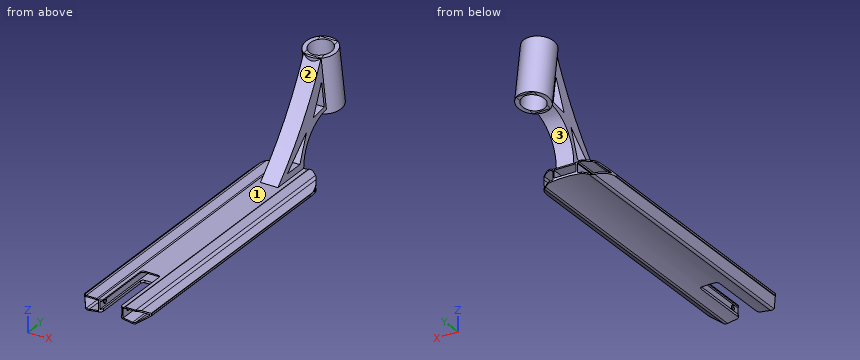
```python
from build123d import *

# Parameters (mm, degrees)
F1_DEPTH       = 250
F2_W           = 38
F2_H           = 13
F3_DEPTH       = 250
F4_T1_DEPTH    = 509.3674969976
F5_R           = 9
F6_R           = 1
F8_DEPTH       = 500.001
F10_DEPTH      = 24.4523840141
F10_DEPTH_BACK = 527
F12_DEPTH      = 527
F12_DEPTH_BACK = 24.4523841141
F13_F1_R       = 4.9999
F13_F2_R       = 4.9999
F13_F3_R       = 5
F13_F4_R       = 5
F13_F5_R       = 5
F13_F6_R       = 5
F15_DEPTH      = 15
F16_R          = 27.4590604355
F17_DEPTH      = 100
F19_D          = 40
F21_D          = 8
F21_DEPTH      = 50
F21_TIP        = 2.4034424761
F23_DEPTH      = 72.5010001


# Not quite as in the source:
# - a fillet or chamfer that OpenCascade refuses, or shapes differently, is made with other operations: its cross-section is extruded or revolved along the edge and cut away or added
# - a fillet or chamfer is up to 0.001 mm smaller than in the source, because OpenCascade refuses the exact size
# - an extrude ends at something that could not be found from the text; its depth is read off the source's solid


with BuildPart() as f1:
    # F0 (on Front) → F1 (new body, symmetric)
    with BuildSketch(Plane.XZ):
        with BuildLine():
            Line((22.5, 23.1513840141), (0, 23.1513840141))
            Line((0, 23.1513840141), (-22.5, 23.1513840141))
            Line((-22.5, 23.1513840141), (-22.5, 24.4513840141))
            Line((-22.5, 24.4513840141), (-45.5824640741, 24.4513840141))
            Line((-45.5824640741, 24.4513840141), (-57.5, 14.4513840141))
            Line((-57.5, 14.4513840141), (-57.5, 10.4513840141))
            Line((-57.5, 10.4513840141), (-40.1794919243, 0.4513840141))
            ThreePointArc((-40.1794919243, 0.4513840141), (0, 4.5289288725), (40.1794919243, 0.4513840141))
            Line((40.1794919243, 0.4513840141), (57.5, 10.4513840141))
            Line((57.5, 10.4513840141), (57.5, 14.4513840141))
            Line((57.5, 14.4513840141), (45.5824640741, 24.4513840141))
            Line((45.5824640741, 24.4513840141), (22.5, 24.4513840141))
            Line((22.5, 24.4513840141), (22.5, 23.1513840141))
        make_face()
    extrude(amount=F1_DEPTH, both=True)

    # F2 (on Front) → F3 (cut, symmetric)
    with BuildSketch(Plane.XZ):
        with Locations((0, 14.6513840141)):
            Rectangle(F2_W, F2_H)
    extrude(amount=F3_DEPTH, both=True, mode=Mode.SUBTRACT)

    # F4: fillet of radius 2 on 2 edges, made by hand

    # F4_s2 → F4_t1 (cut)
    with BuildSketch(Plane.XZ.offset(-254.6837484988)):
        with BuildLine():
            ThreePointArc((-24.3734993995, 24.4513840141), (-23.2333239744, 24.0945516866), (-22.5, 23.1513840141))
            Line((-22.5, 23.1513840141), (-22.5, 24.4513840141))
            Line((-22.5, 24.4513840141), (-24.3734993995, 24.4513840141))
        make_face()
        with BuildLine():
            ThreePointArc((24.3734993995, 24.4513840141), (23.2333239744, 24.0945516866), (22.5, 23.1513840141))
            Line((22.5, 23.1513840141), (22.5, 24.4513840141))
            Line((22.5, 24.4513840141), (24.3734993995, 24.4513840141))
        make_face()
    extrude(amount=F4_T1_DEPTH, mode=Mode.SUBTRACT)

    # F5
    f5_edges = [f1.edges().sort_by_distance(p)[0] for p in [
        (-45.582464, 0, 24.451384),
        (-40.179492, 0, 0.451384),
        (40.179492, 0, 0.451384),
        (45.582464, 0, 24.451384),
    ]]
    fillet(f5_edges, radius=F5_R)

    # F6
    f6_edges = [f1.edges().sort_by_distance(p)[0] for p in [
        (57.5, 0, 14.451384),
        (57.5, 0, 10.451384),
        (-57.5, 0, 10.451384),
        (-57.5, 0, 14.451384),
    ]]
    fillet(f6_edges, radius=F6_R)

    # F7 (on face) → F8 (cut, through all)
    with BuildSketch(Plane.XZ.offset(250)):
        with BuildLine():
            ThreePointArc((-42.1022690923, 3.8709010064), (-39.7790673433, 3.0327059534), (-37.3093701274, 3.0535140017))
            ThreePointArc((-37.3093701274, 3.0535140017), (-29.1789785809, 4.4103617496), (-21, 5.4343792715))
            Line((-21, 5.4343792715), (-21, 21.1513840141))
            Line((-21, 21.1513840141), (-22.5, 21.1513840141))
            ThreePointArc((-22.5, 21.1513840141), (-23.2333239744, 22.0945516866), (-24.3734993995, 22.4513840141))
            Line((-24.3734993995, 22.4513840141), (-42.3067319657, 22.4513840141))
            ThreePointArc((-42.3067319657, 22.4513840141), (-44.7008729689, 22.0292323596), (-46.8062452335, 20.813695116))
            Line((-46.8062452335, 20.813695116), (-55.7563117574, 13.3036975967))
            ThreePointArc((-55.7563117574, 13.3036975967), (-56.1097188459, 12.4504974108), (-55.6135241478, 11.6716277498))
            Line((-55.6135241478, 11.6716277498), (-42.1022690923, 3.8709010064))
        make_face()
        with BuildLine():
            Line((21, 21.1513840141), (21, 5.4343792715))
            ThreePointArc((21, 5.4343792715), (29.1789785809, 4.4103617496), (37.3093701274, 3.0535140017))
            ThreePointArc((37.3093701274, 3.0535140017), (39.7790673433, 3.0327059534), (42.1022690923, 3.8709010064))
            Line((42.1022690923, 3.8709010064), (55.6135241478, 11.6716277498))
            ThreePointArc((55.6135241478, 11.6716277498), (56.1097188459, 12.4504974108), (55.7563117574, 13.3036975967))
            Line((55.7563117574, 13.3036975967), (46.8062452335, 20.813695116))
            ThreePointArc((46.8062452335, 20.813695116), (44.7008729689, 22.0292323596), (42.3067319657, 22.4513840141))
            Line((42.3067319657, 22.4513840141), (24.3734993995, 22.4513840141))
            ThreePointArc((24.3734993995, 22.4513840141), (23.2333239744, 22.0945516866), (22.5, 21.1513840141))
            Line((22.5, 21.1513840141), (21, 21.1513840141))
        make_face()
    extrude(amount=-F8_DEPTH, mode=Mode.SUBTRACT)

    # F9 (on Top) → F10 (cut, two sides)
    with BuildSketch(Plane.XY) as f10_sk:
        with BuildLine():
            ThreePointArc((-57.5, 200), (0, 257.5), (57.5, 200))
            Line((57.5, 200), (57.5, 280))
            Line((57.5, 280), (-57.5, 280))
            Line((-57.5, 280), (-57.5, 200))
        make_face()
    extrude(amount=F10_DEPTH, mode=Mode.SUBTRACT)
    extrude(f10_sk.sketch, amount=-F10_DEPTH_BACK, mode=Mode.SUBTRACT)

    # F11 (on Top) → F12 (cut, two sides)
    with BuildSketch(Plane.XY) as f12_sk:
        Polygon((-43.2975540478, -250), (-68, -216), (-68, -346), (68, -346), (68, -216), (43.2975540478, -250), (16, -250), (16, -140), (-16, -140), (-16, -250), align=None)
    extrude(amount=-F12_DEPTH, mode=Mode.SUBTRACT)
    extrude(f12_sk.sketch, amount=F12_DEPTH_BACK, mode=Mode.SUBTRACT)

    # F13: fillet of radius 5 on 8 edges, made by hand

    # F13_f1 (radius 5 in the source; OpenCascade refuses exactly that, so slightly less here)
    f13_f1_edges = [f1.edges().sort_by_distance(p)[0] for p in [
        (-16, -250, 22.1513840141),
    ]]
    fillet(f13_f1_edges, radius=F13_F1_R)

    # F13_f2 (radius 5 in the source; OpenCascade refuses exactly that, so slightly less here)
    f13_f2_edges = [f1.edges().sort_by_distance(p)[0] for p in [
        (16, -250, 6.0196427984),
    ]]
    fillet(f13_f2_edges, radius=F13_F2_R)

    # F13_f3
    f13_f3_edges = [f1.edges().sort_by_distance(p)[0] for p in [
        (16, -140, 22.1513840141),
    ]]
    fillet(f13_f3_edges, radius=F13_F3_R)

    # F13_f4
    f13_f4_edges = [f1.edges().sort_by_distance(p)[0] for p in [
        (-16, -140, 22.1513840141),
    ]]
    fillet(f13_f4_edges, radius=F13_F4_R)

    # F13_f5
    f13_f5_edges = [f1.edges().sort_by_distance(p)[0] for p in [
        (-16, -140, 6.0196427984),
    ]]
    fillet(f13_f5_edges, radius=F13_F5_R)

    # F13_f6
    f13_f6_edges = [f1.edges().sort_by_distance(p)[0] for p in [
        (16, -140, 6.0196427984),
    ]]
    fillet(f13_f6_edges, radius=F13_F6_R)

    # F14 (on Right) → F15 (join, symmetric)
    with BuildSketch(Plane.YZ):
        with BuildLine():
            ThreePointArc((297.3819995028, 183.1513840141), (245.9666940414, 97.8136618671), (180, 23.1513840141))
            Line((180, 23.1513840141), (250, 23.1513840141))
            ThreePointArc((250, 23.1513840141), (267.6550746197, 69.6272787008), (311.7145367693, 92.6593051387))
            Line((311.7145367693, 92.6593051387), (313.0254460068, 84.3825499546))
            Line((313.0254460068, 84.3825499546), (358.4591096742, 91.5785353465))
            Line((358.4591096742, 91.5785353465), (342.8156631702, 190.347369406))
            Line((342.8156631702, 190.347369406), (297.3819995028, 183.1513840141))
        make_face()
    extrude(amount=F15_DEPTH, both=True)

    # F16 (on face) → F17 (join, through all)
    with BuildSketch(Plane(origin=(0, -21.0209895784, 132.7213047908), x_dir=(1, 0, 0), z_dir=(0, -0.156434465, 0.9876883406))):
        with Locations((0, 345.3719223914)):
            Circle(F16_R)
    extrude(amount=-F17_DEPTH)

    # F19 (through all)
    with Locations(Plane(origin=(0, -21.0209895784, 132.7213047908), x_dir=(1, 0, 0), z_dir=(0, -0.156434465, 0.9876883406))):
        with Locations((0, 345.3719223914)):
            Hole(F19_D / 2)

    # F21 (one way)
    with BuildSketch(Plane.YZ.offset(21)):
        with Locations((-236, 15.4343792715)):
            Circle(F21_D / 2)
    extrude(amount=-F21_DEPTH, mode=Mode.SUBTRACT)
    with Locations(Plane.YZ.offset(21)):
        with Locations((-236, 15.4343792715)):
            with Locations((0, 0, -(F21_DEPTH + F21_TIP / 2))):  # 118° drill point
                Cone(0, F21_D / 2, F21_TIP, mode=Mode.SUBTRACT)

    # F22 (on face) → F23 (cut, through all)
    with BuildSketch(Plane.YZ.offset(15)):
        Polygon((205.6868169308, 34.2114791274), (239.6868169308, 33.9609570801), (257.5687806787, 78.9609570801), align=None)
        Polygon((305.8015852264, 98.9295560122), (298.6742854118, 143.9295560122), (276.1709350086, 94.2365220609), align=None)
    extrude(amount=-F23_DEPTH, mode=Mode.SUBTRACT)


solid = f1.part
```
Source: CAD feature listing. Evaluate the final solid. Frame: model axes, mm. Face numbers are marked on the shaded views. Coordinates: 2 decimals unless noted, no trailing zeros. Loops run counter-clockwise (first coordinate to the right, second up) from the corner with the lowest first, then second, coordinate; pieces in that order, holes last. Notation, with made-up numbers: M 48.25,-35.5 L 79.25,-35.5 A23 cw 79.25,-6.5 Z; hole C -29.5,23.5 d8. An arc over 180 degrees is marked long. Use a Markdown table: item, result. Add a question column.
Q1. First-contact query: pin 1 (3 mm diameter, centred on y = 74, z = 23.5, fed in from +X); pin 2 (1.2 mm diameter, centred on x = 21.5, y = 78, fed in from -Z); pin 3 (5 mm diameter, centred on y = -236, z = 15.43, fed in from +X); pin 4 (17.5 mm diameter, centred on y = -34, z = 16.5, fed in from +X). Flat tips, straight axial feed; report the tip coordinate or a pass-through.
Q2. Material intervals for L1, parallel to Z at x = -20.2, y = -236; L2, parallel to Z at x = 30, y = 212; L3, parallel to Z at x = 14, y = 228, sorted ascending.
Q3. Draft query along Y for the marked faces 1, 2 and 3. Return one class per face: pulls with the +Y half, pulls with the -Y half, needs draft (parallel to the pull), parting line crosses it, or undercut.
Q4. Section query B-B, the plane y = -166.5. State how many separate pieces and enclosed holes the cut face has, and give its area (3 significant figures).
Q5. Section query A-A, the plane x = 5.5. Return loops of the section in (y, z), and give its area (3 significant figures).
Q6. Section query C-C, the plane z = 53.5. Return loops of the section in (x, y), and give its area (3 significant figures).
Result:
| question | item | result |
|---|---|---|
| 1 | pin 1 | stops at x = 48.5 |
| 1 | pin 2 | stops at z = 3.3 |
| 1 | pin 3 | stops at x = 55.29 |
| 1 | pin 4 | stops at x = 57.5 |
| 2 | L1 | z = 3.51 to 11.43, 19.43 to 23.15 |
| 2 | L2 | z = 2.27 to 4.29, 22.45 to 24.45 |
| 2 | L3 | z = 4.04 to 8.15, 21.15 to 34.05, 53.46 to 74.64 |
| 3 | face 1 | needs draft |
| 3 | face 2 | pulls with the -Y half |
| 3 | face 3 | undercut |
| 4 | separate pieces | 2 |
| 4 | enclosed holes | 2 |
| 4 | area | 434 mm2 |
| 5 | outline | M -140,4.45 L 250,4.45 L 250,8.15 L -140,8.15 Z; M -140,21.15 L 250,21.15 L 250,23.15 A70 cw 307.85,92.09 L 309.17,83.77 L 316.75,84.97 L 301.11,183.74 L 293.53,182.54 L 294.39,177.08 A550 cw 180,23.15 L -140,23.15 Z; M 339.09,189.76 L 354.73,90.99 L 362.31,92.19 L 346.67,190.96 Z; hole M 205.69,34.21 L 239.69,33.96 L 257.57,78.96 Z; hole M 276.17,94.24 L 305.8,98.93 L 298.67,143.93 Z |
| 5 | area | 8,530 mm2 |
| 6 | outline | M -15,209.76 L 15,209.76 L 15,228.05 L -15,228.05 Z; M -15,247.45 L 15,247.45 L 15,256.92 L -15,256.92 Z |
| 6 | area | 833 mm2 |
